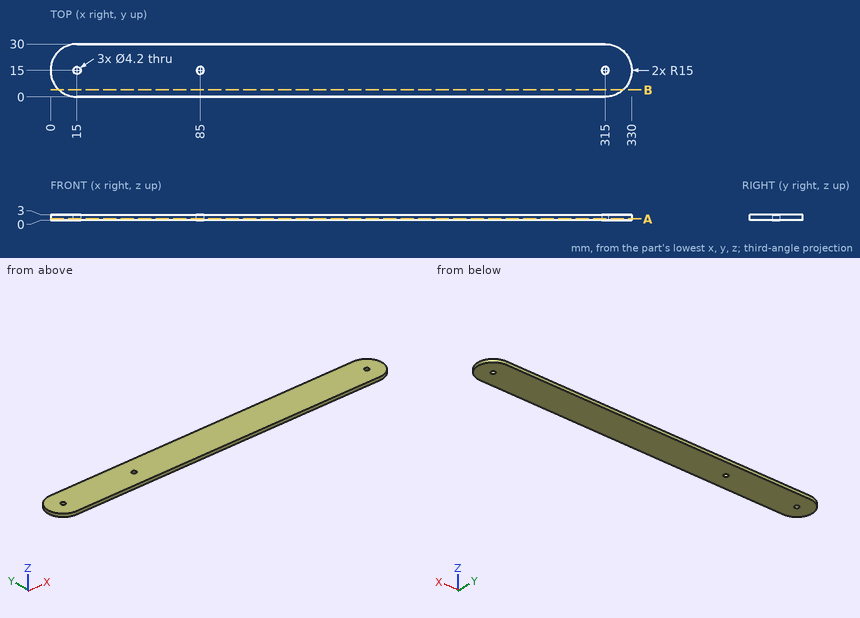
Design review of the part shown in the three views and the two pictorial views. Dimensions are in mm from the part's minimum x, y and z. Give positions to 0.01 mm unless a question says otherwise; leave off trailing zeros. Write each loop counter-clockwise with the first axis right and the second up, starting at its lowest first coordinate (ties: lowest second). Pieces come first, ordered by that corner, then holes. Notation, with made-up numbers: M -28,32 L -16,32 A18 cw -16,43 Z; hole C 10.25,-26 d10. An arc over 180 degrees is marked long. Answer in a Markdown table with one row per item.
Item 1: For line 1 along X through (y, z) = (14.75, 2.05); line 2 along Y through (x, z) = (315, 1.45); line 3 along X through (y, z) = (2, 0.9), list the stretches that pass through material, from the lowest coordinate up.
Check sheet entries:
| item | result |
|---|---|
| line 1 | 0 to 12.91, 17.09 to 82.91, 87.09 to 312.91, 317.09 to 330 |
| line 2 | 0 to 12.9, 17.1 to 30 |
| line 3 | 7.52 to 322.48 |
Item 2: Add section B-B on y = 4. Give the boundary of the cut face in (x, z).
Check sheet entries:
| item | result |
|---|---|
| outline | M 4.8,0 L 325.2,0 L 325.2,3 L 4.8,3 Z |
Item 3: Add section A-A on z = 0.65. Give the boundary of the cut face in (x, y).
Check sheet entries:
| item | result |
|---|---|
| outline | M 15,0 L 315,0 A15 ccw 315,30 L 15,30 A15 ccw Z; hole C 15,15 d4.2; hole C 85,15 d4.2; hole C 315,15 d4.2 |
Item 4: For P1, Ø5.5, axis at x = 15, y = 15, coming from the -Z side; P2, Ø1, axis at y = 25, z = 0.5, coming from the +X side; P3, Ø1, axis at y = 23, z = 1, coming from the +X side, all flat-tipped, find the tip position at first contact; note any pin that passes through.
Check sheet entries:
| item | result |
|---|---|
| P1 | z = 0 |
| P2 | x = 326.61 |
| P3 | x = 327.99 |
